Geometry: final body of the model. Coordinates: model frame, mm. Give positions to 0.01 mm unless a question says otherwise; leave off trailing zeros. Write each loop counter-clockwise with the first axis right and the second up, starting at its lowest first coordinate (ties: lowest second). Pieces come first, ordered by that corner, then holes. Notation, with made-up numbers: M 59,53 L 91,53 A15 cw 91,69 Z; hole C -10,-35 d1. An arc over 180 degrees is marked long. Use one line per item in the form item = value. Start each with the question number.
Item 1: Contact query for flat-ended pins moving along their axis: P1, Ø5.5, axis at x = -82.5, y = -32.5, coming from the -Z side; P2, Ø9, axis at x = 82.5, y = 32.5, coming from the +Z side. Output: stop coordinate, or through.
Item 2: Section query B-B on x = 82.5. Return loops of the section in (y, z).
Item 3: Section query C-C on z = 0.4. Return loops of the section in (x, y).
Item 4: Section query A-A on y = 32.5. Return loops of the section in (x, z), then the cut area to 3 significant figures.
Item 5: Section query D-D on x = 0. Return loops of the section in (y, z), then the cut area to 3 significant figures.
Item 6: Material intervals for line 1 along Y through (x, z) = (0, 0.3); line 2 along Y through (x, z) = (82.5, 0.85); line 3 along X through (y, z) = (14, 0.9), sorted ascending. Write a range as from..to.
from build123d import *

# Parameters (mm, degrees)
SKETCH1_W                = 179
SKETCH1_H                = 79
BOSS_EXTRUDE1_DEPTH      = 1
FILLET1_R                = 3
F_7_0_7_DIAMETER_HOLE1_D = 7
SKETCH4_W                = 155
SKETCH4_H                = 53
CUT_EXTRUDE1_DEPTH       = 98.834043155
FILLET2_R                = 3


with BuildPart() as part:
    # Sketch1 → Boss-Extrude1 (new body)
    with BuildSketch(Plane.XY):
        Rectangle(SKETCH1_W, SKETCH1_H)
    extrude(amount=BOSS_EXTRUDE1_DEPTH)

    # Fillet1
    fillet1_edges = [part.edges().sort_by_distance(p)[0] for p in [
        (89.5, -39.5, 0.5),
        (-89.5, -39.5, 0.5),
        (-89.5, 39.5, 0.5),
        (89.5, 39.5, 0.5),
    ]]
    fillet(fillet1_edges, radius=FILLET1_R)

    # Ø7.0 (7) Diameter Hole1 (through all)
    with Locations(Plane.XY.offset(1)):
        with Locations((0, 32.5), (-82.5, 32.5), (82.5, 32.5), (82.5, -32.5), (0, -32.5), (-82.5, -32.5)):
            Hole(F_7_0_7_DIAMETER_HOLE1_D / 2)

    # Sketch4 → Cut-Extrude1 (cut, through all)
    with BuildSketch(Plane.XY.offset(1)):
        Rectangle(SKETCH4_W, SKETCH4_H)
    extrude(amount=-CUT_EXTRUDE1_DEPTH, mode=Mode.SUBTRACT)

    # Fillet2
    fillet2_edges = [part.edges().sort_by_distance(p)[0] for p in [
        (-77.5, -26.5, 0.5),
        (-77.5, 26.5, 0.5),
        (77.5, 26.5, 0.5),
        (77.5, -26.5, 0.5),
    ]]
    fillet(fillet2_edges, radius=FILLET2_R)


solid = part.part
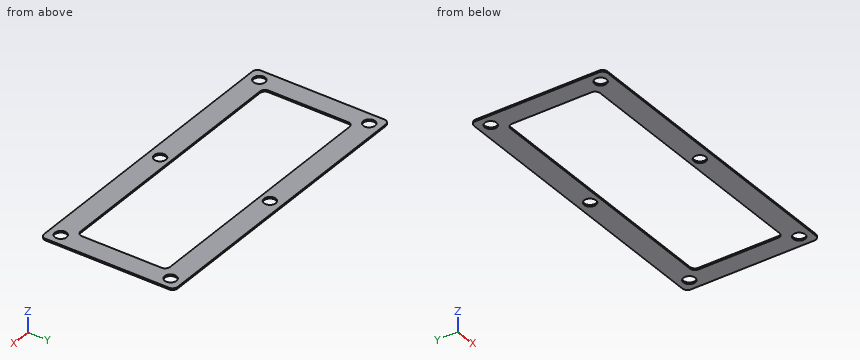
Answer sheet:
q1.P1 = through
q1.P2 = 1
q2.outline = M -39.5,0 L -36,0 L -36,1 L -39.5,1 Z; M -29,0 L 29,0 L 29,1 L -29,1 Z; M 36,0 L 39.5,0 L 39.5,1 L 36,1 Z
q3.outline = M -89.5,-36.5 A3 ccw -86.5,-39.5 L 86.5,-39.5 A3 ccw 89.5,-36.5 L 89.5,36.5 A3 ccw 86.5,39.5 L -86.5,39.5 A3 ccw -89.5,36.5 Z; hole C -82.5,-32.5 d7; hole C -82.5,32.5 d7; hole M -77.5,-23.5 A3 ccw -74.5,-26.5 L 74.5,-26.5 A3 ccw 77.5,-23.5 L 77.5,23.5 A3 ccw 74.5,26.5 L -74.5,26.5 A3 ccw -77.5,23.5 Z; hole C 0,-32.5 d7; hole C 0,32.5 d7; hole C 82.5,-32.5 d7; hole C 82.5,32.5 d7
q4.outline = M -89.5,0 L -86,0 L -86,1 L -89.5,1 Z; M -79,0 L -3.5,0 L -3.5,1 L -79,1 Z; M 3.5,0 L 79,0 L 79,1 L 3.5,1 Z; M 86,0 L 89.5,0 L 89.5,1 L 86,1 Z
q4.area = 158 mm2
q5.outline = M -39.5,0 L -36,0 L -36,1 L -39.5,1 Z; M -29,0 L -26.5,0 L -26.5,1 L -29,1 Z; M 26.5,0 L 29,0 L 29,1 L 26.5,1 Z; M 36,0 L 39.5,0 L 39.5,1 L 36,1 Z
q5.area = 12.0 mm2
q6.line_1 = -39.5..-36, -29..-26.5, 26.5..29, 36..39.5
q6.line_2 = -39.5..-36, -29..29, 36..39.5
q6.line_3 = -89.5..-77.5, 77.5..89.5
